Autodesk Fusion 360 part; units mm, degrees
sphere "SpherePrimitive1" add diameter 40 placed x (0, 1, 0) y (0, 0, 1) z (1, 0, 0) at (0, 0, 0)
cylinder "CylindrePrimitive1" add diameter 8 height 30 placed x (0, 0, -1) y (0, 1, 0) z (1, 0, 0) at (0, 0.2086, 0)
cylinder "CylindrePrimitive2" add diameter 3 height 4 placed x (0, 0, -1) y (0, 1, 0) z (1, 0, 0) at (30, 0, 0)
thread "Filetage1" thread offset 0 thread length 10
Design review of the part built by this model. Coordinates are the model's own, in mm. Give positions to 0.01 mm unless a question says otherwise; leave off trailing zeros. Loops run counter-clockwise (first coordinate to the right, second up) from the corner with the lowest first, then second, coordinate; pieces in that order, holes last. Notation, with made-up numbers: (34.25, -6.5) - (55.25, -6.5) arc R22 cw to (55.25, 5.5) - close; hole circle Ø1 at (-22, 16.25). An arc over 180 degrees is marked (long way). Write item = value, one per line.
1) Take a section at B-B on x = 17. State the section outline as (y, z) points, and give its area (3 significant figures).
Result sheet:
outline = circle Ø21.07 at (0, 0)
area = 349 mm2
2) To check wall thickness, follow line 1 (X direction, y = -1.5, z = -11.5); line 2 (X direction, y = -17, z = -3); line 3 (Z direction, x = -3.5, y = -4). State the ranges of each line that lie inside material, in increasing order.
Result sheet:
line_1 = -16.29 to 16.29
line_2 = -10.1 to 10.1
line_3 = -19.28 to 19.28
3) Take a section at C-C on y = 13.5. State the section outline as (x, z) points, and give its area (3 significant figures).
Result sheet:
outline = circle Ø29.51 at (0, 0)
area = 684 mm2
4) Take a section at A-A on z = 0. State the section outline as (x, y) points, and give its area (3 significant figures).
Result sheet:
outline = (19.55, 4.21) arc R20 ccw (long way) to (19.64, -3.79) - (30, -3.79) - (30, -1.5) - (34, -1.5) - (34, 1.5) - (30, 1.5) - (30, 4.21) - close
area = 1,350 mm2
5) Draft analysis for pull direction X (two halves, no side actions). For faces 1 (the face through (32.03, 0.07, 1.5)), 2 (the face through (34, 0, 0)), state which applies: +X half, -X half, draft (parallel to the pull), parting line (faces both ways), or undercut.
Result sheet:
face_1 = draft
face_2 = +X half
6) Clearance check with flat-ended pins moving along their axes: pin 1 Ø1.5 at (x, z) = (-4, 11) entering from -Y; pin 2 Ø4 at (x, y) = (28, 0) entering from +Z; pin 3 Ø3 at (y, z) = (2.5, 8.5) entering from +X. State where each tip first meets the part, or that it passes through.
Result sheet:
pin_1 = -16.73
pin_2 = 4
pin_3 = 18.6
